Check sheet for the modelled part. Datum: model origin and axes. Units: mm. A direction names the side the tool comes from. Give positions to 0.01 mm unless a question says otherwise; leave off trailing zeros. Write item = value, one per line. Start each with the question number.
1) Scan lines: line 1 along Z through (x, y) = (0, -12.9); line 2 along X through (y, z) = (-14.1, 6.35); line 3 along X through (y, z) = (-9.5, 3.5). Record each from-to range of solid material in increasing order. Write a range as [from, to].
2) Mould release check, pull along Z, two halves, no side actions. Record for faces 1 (the flat face through (-2.2, -0.2, 0)), 2 (the flat face through (27.4, -6.8, 6.3)), 3 (the cylindrical face through (-20.144, -4.632, 6.251)): released by +Z, released by -Z, zero draft, split by the parting line, or undercut.
3) Access from +Z, -Z, +X, -X, +Y, -Y to the whole of each face (thin tool, end or side, straight path). Record for faces 4 (the flat face through (-27.4, -6.8, 6.3)), 5 (the cylindrical face through (0, -13, 8)), 6 (the flat face through (-1, -11.481, 8)), 7 (the cylindrical face through (-20.147, -6.292, 6.275)), 8 (the flat face through (-2.2, -0.2, 12.7)).
4) Cross-section at A-A, the plane x = 0. Give the number of separate pieces and of enclosed holes in the cut face, plus the area to 3 significant figures.
5) Go/stop test with flat-tipped pins: pin 1 (2 mm diameter, centred on x = -3, z = 2, fed in from -Y); pin 2 (1 mm diameter, centred on x = -16, z = 1.5, fed in from +Y); pin 3 (3 mm diameter, centred on x = 0, z = 6.35, fed in from +Y). Record where each tip stops, or that it passes through.
```python
from build123d import *

# Parameters (mm, degrees)
BOSS_EXTRUDE1_DEPTH = 12.7
SKETCH2_R           = 1.651
CUT_EXTRUDE1_DEPTH  = 33.458037303
SKETCH4_R           = 2.25298
CUT_EXTRUDE3_DEPTH  = 34.719236888
FILLET1_R           = 2
FILLET2_R           = 1
CUT_EXTRUDE4_DEPTH  = 34.974608094


with BuildPart() as part:
    # Sketch1 → Boss-Extrude1 (new body)
    with BuildSketch(Plane.XY):
        with BuildLine():
            Line((-27.839103255, -5.787477181), (-26.57368947, -8.699410036))
            ThreePointArc((-26.57368947, -8.699410036), (-17.565333038, -5.530370801), (-8.196652556, -3.680743454))
            ThreePointArc((-8.196652556, -3.680743454), (0, -14.76375), (8.196652556, -3.680743454))
            ThreePointArc((8.196652556, -3.680743454), (17.565333038, -5.530370801), (26.57368947, -8.699410036))
            Line((26.57368947, -8.699410036), (27.839103255, -5.787477181))
            ThreePointArc((27.839103255, -5.787477181), (0, 0), (-27.839103255, -5.787477181))
        make_face()
        with BuildLine():
            Line((-2.764985714, -10.82675), (2.764985714, -10.82675))
            ThreePointArc((2.764985714, -10.82675), (0, -0.79375), (-2.764985714, -10.82675))
        make_face(mode=Mode.SUBTRACT)
    extrude(amount=BOSS_EXTRUDE1_DEPTH)

    # Sketch2 → Cut-Extrude1 (cut, through all)
    with BuildSketch(Plane(origin=(0, -10.82675, 0), x_dir=(1, 0, 0), z_dir=(0, 1, 0))):
        with Locations(Location((0, -6.35, 0), (0, 0, 270))):
            Circle(SKETCH2_R)
    extrude(amount=-CUT_EXTRUDE1_DEPTH, mode=Mode.SUBTRACT)

    # Sketch4 → Cut-Extrude3 (cut, through all)
    with BuildSketch(Plane(origin=(0.366542573, -1.342182486, 0), x_dir=(0.9646738537497861, 0.2634470646857473, 0), z_dir=(-0.2634470646857473, 0.9646738537497861, 0))):
        with Locations((-18.401777468, -6.35)):
            Circle(SKETCH4_R)
    cut_extrude3 = extrude(amount=CUT_EXTRUDE3_DEPTH, mode=Mode.SUBTRACT)

    # Mirror1: Cut-Extrude3 across plane
    add(cut_extrude3.mirror(Plane(origin=(0, 0, 0), x_dir=(0, 0, 1), z_dir=(1, 0, 0))), mode=Mode.SUBTRACT)

    # Fillet1
    fillet1_edges = [part.edges().sort_by_distance(p)[0] for p in [
        (8.196652556, -3.680743454, 6.35),
        (-8.196652556, -3.680743454, 6.35),
    ]]
    fillet(fillet1_edges, radius=FILLET1_R)

    # Fillet2
    fillet2_edges = [part.edges().sort_by_distance(p)[0] for p in [
        (26.57368947, -8.699410036, 6.35),
        (-26.57368947, -8.699410036, 6.35),
        (-18.878378383, -5.903440635, 12.7),
        (0, -14.76375, 0),
        (0, -14.76375, 12.7),
        (18.878378383, -5.903440635, 0),
        (18.878378383, -5.903440635, 12.7),
        (-9.267474809, -4.528405008, 0),
        (-9.267474809, -4.528405008, 12.7),
        (9.267474809, -4.528405008, 0),
        (9.267474809, -4.528405008, 12.7),
        (-18.878378383, -5.903440635, 0),
    ]]
    fillet(fillet2_edges, radius=FILLET2_R)

    # Sketch5 → Cut-Extrude4 (cut, through all)
    with BuildSketch(Plane.XY.offset(12.7)):
        with BuildLine():
            Line((-3.155336639, -11.481173529), (3.155336639, -11.481173529))
            ThreePointArc((3.155336639, -11.481173529), (0, -0.03175), (-3.155336639, -11.481173529))
        make_face()
    extrude(amount=-CUT_EXTRUDE4_DEPTH, mode=Mode.SUBTRACT)


solid = part.part
```
Reply:
q1.line_1 = [0, 4.7], [8, 12.7]
q1.line_2 = [-3.31, -1.65], [1.65, 3.31]
q1.line_3 = [-7.91, -5.2], [5.2, 7.91]
q2.face_1 = released by -Z
q2.face_2 = zero draft
q2.face_3 = undercut
q3.face_4 = +Z, -Z, -X, -Y
q3.face_5 = -Y
q3.face_6 = +Z, -Z
q3.face_7 = +Z, -Z, -Y
q3.face_8 = +Z, +X, -X, +Y, -Y
q4.separate_pieces = 3
q4.enclosed_holes = 0
q4.area = 30.8 mm2
q5.pin_1 = -14.53
q5.pin_2 = -1.74
q5.pin_3 = 0
